Input: part model. Units: mm. Frame: model coordinates. Face numbers are marked on the shaded views. A direction names the side the tool comes from. Round coordinates to 2 decimals unless told otherwise and drop trailing zeros. Order: outer loops, then holes, each group sorted by start corner. A loop starts at its lowest first (then second) coordinate and runs counter-clockwise, first axis right, second up. Notation, with made-up numbers: M 71.5,5.25 L 129.5,5.25 A24 cw 129.5,33.25 Z; hole C -11,-9.5 d5. An arc over 180 degrees is marked long. One line per question, with ' | ' between items.
```python
from build123d import *

# Parameters (mm, degrees)
RESSALTO_EXTRUS_O1_DEPTH = 6.5
ESBO_O4_R                = 1.5
CORTE_EXTRUS_O1_DEPTH    = 31.317074397


with BuildPart() as part:
    # Esboço1 → Revolução1 (revolve)
    with BuildSketch(Plane.XY):
        Polygon((0, 0), (-19.5, 0), (-19.5, 6.25), (-11, 6.25), (-11, 4), (-9, 4), (-8, 5), (-1, 5), (0, 4), align=None)
    revolve(axis=Axis((0, 0, 0), (-1, 0, 0)))

    # Esboço2 → Ressalto-extrusão1 (add)
    with BuildSketch(Plane.ZY.offset(19.5)):
        Polygon((-5.5, 2.968585522), (-5.5, -2.968585522), (0, -6.25), (5.5, -2.968585522), (5.5, 2.968585522), (0, 6.25), align=None)
    extrude(amount=RESSALTO_EXTRUS_O1_DEPTH)

    # Esboço3 → Revolução2 (revolve)
    with BuildSketch(Plane.XY, mode=Mode.PRIVATE) as revolu_o2_sk:
        Polygon((-29, 0), (-26, 0), (-26, 4), (-28, 4), (-29, 5), (-36, 5), (-37, 4), (-37, 2.5), (-29.707106781, 2.5), (-29, 1.792893219), align=None)
    revolve(revolu_o2_sk.sketch.rotate(Axis((-29, 0, 0), (1, 0, 0)), 180), axis=Axis((-29, 0, 0), (1, 0, 0)))

    # Esboço4 → Corte-extrusão1 (cut, through all)
    with BuildSketch(Plane.ZY.offset(29)):
        with Locations(Location((0, 0, 0), (0, 0, 270))):
            Circle(ESBO_O4_R)
    extrude(amount=-CORTE_EXTRUS_O1_DEPTH, mode=Mode.SUBTRACT)


solid = part.part
```
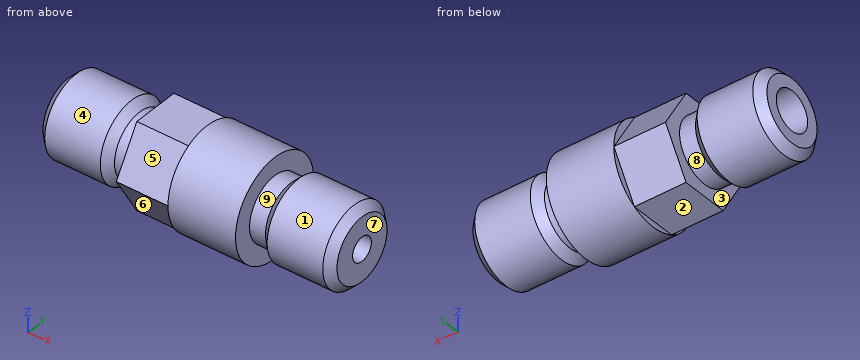
Item 1: Section query B-B, the plane y = 4.5. Give the number of separate pieces and of enclosed holes in the cut face, plus the area to 3 significant figures.
Report:
separate pieces: 3 | enclosed holes: 0 | area: 179 mm²
Item 2: Line query: line 1 along Z through (x, y) = (-32.5, 0); line 2 along X through (y, z) = (2, 4.25); line 3 along X through (y, z) = (-0.75, -4.75). Output: solid intervals per line, ascending. Write a range as from..to.
Report:
line 1: -5..-2.5, 2.5..5 | line 2: -36.3..-28.7, -26..-11, -8.3..-0.7 | line 3: -36.19..-28.81, -26..-11, -8.19..-0.81
Item 3: Section query D-D, the plane x = -28.5. Return loops of the section in (y, z).
Report:
outline: C 0,0 d9; hole C 0,0 d3
Item 4: Section query C-C, the plane y = -5.5. Return loops of the section in (x, z), plus the area to 3 significant figures.
Report:
outline: M -26,-1.26 L -19.5,-1.26 L -19.5,-2.97 L -11,-2.97 L -11,2.97 L -19.5,2.97 L -19.5,1.26 L -26,1.26 Z | area: 66.8 mm²
Item 5: Access query for the marked faces 1, 2, 3, 4 and 5. Directions: +Z, -Z, +X, -X, +Y, -Y. A direction counts if a zero-diameter tool reaches every point of the face in a straight line with its end or side. Return the directions, or none.
Report:
face 1: +X | face 2: -Z, -X, +Y, -Y | face 3: none | face 4: -X | face 5: +Z, -X, -Y
Item 6: Section query A-A, the plane x = -15. Return loops of the section in (y, z), plus the area to 3 significant figures.
Report:
outline: C 0,0 d12.5; hole C 0,0 d3 | area: 116 mm²
Item 7: Mould query, pull axis X, two halves, no side actions, for the marked faces 6, 7, 8 and 9. Classes: +X half, -X half, draft (parallel to the pull), parting line (faces both ways), or undercut.
Report:
face 6: draft | face 7: +X half | face 8: undercut | face 9: undercut
Item 8: First-contact query: pin 1 (6 mm diameter, centred on y = 0, z = 0, fed in from -X); pin 2 (4.5 mm diameter, centred on x = -21.5, y = 1.5, fed in from +Z); pin 3 (2.5 mm diameter, centred on y = -4.5, z = 3, fed in from -X); pin 4 (2 mm diameter, centred on x = -7.5, y = -4.5, fed in from -Z). Flat tips, straight axial feed; report the tip coordinate or a pass-through.
Report:
pin 1: x = -37 | pin 2: z = 6.23 | pin 3: x = -36.84 | pin 4: z = -3.57
